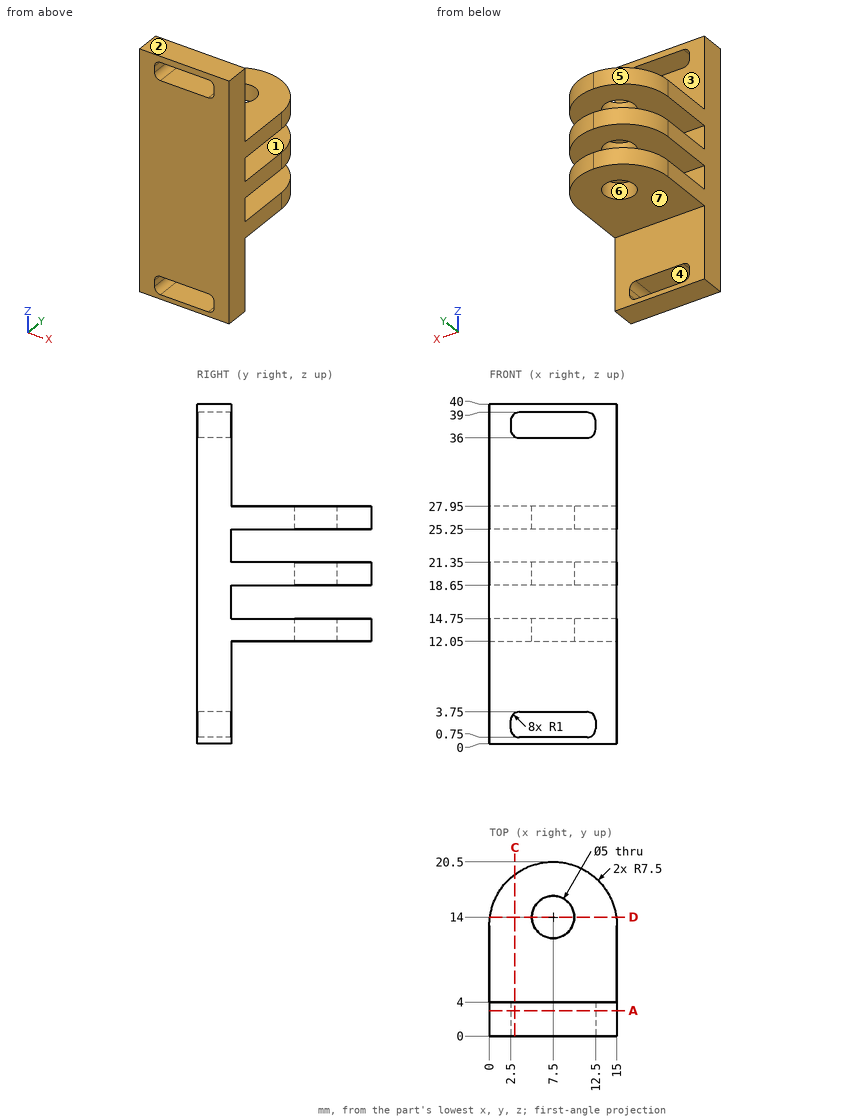
Here's the drawing with two shaded views (mm, measured from the low corner). I have some questions. A direction names the side the tool comes from. Coordinates: 2 decimals unless noted, no trailing zeros. Write each loop counter-clockwise with the first axis right and the second up, starting at its lowest first coordinate (ties: lowest second). Pieces come first, ordered by that corner, then holes. Notation, with made-up numbers: M 36.5,39 L 90.5,39 A26 cw 90.5,78 Z; hole C 54,18 d5. An arc over 180 degrees is marked long. Answer as CSV lines item,"result". Start each with the question number.
1) I want a section at A-A, the plane y = 3. Please give me the cut outline in (x, z), and give its area (3 significant figures).
2) I want a section at D-D, the plane y = 14. Please give me the cut outline in (x, z).
3) Please list where these lines run through material, in increasing order: line 1 (Z direction, x = 10.75, y = 11.25); line 2 (Y direction, x = 7.5, z = 19.3); line 3 (Y direction, x = 6.75, z = 8.5). Write a range as from..to.
4) For P1, Ø1.2, axis at x = 6, z = 24, coming from the +Y side; P2, Ø4, axis at x = 9.5, y = 14.5, coming from the +Z side; P3, Ø5, axis at x = 3.5, y = 14, coming from the -Z side, each with a flat end and sliding along its axis, tell me the tip position at first contact or that it passes through.
5) For the marked faces 1, 2, 3 and 4, which set-ups out of +Z, -Z, +X, -X, +Y, -Y let a thin tool reach every point of the face, with its end or its side?
6) I want a section at C-C, the plane x = 3. Please give me the cut outline in (y, z).
7) We'd pull the mould along X, two halves only. Please class the marked faces 5, 6 and 7: +X half, -X half, draft (parallel to the pull), parting line (faces both ways), or undercut.
Data:
1,outline,"M 0,0 L 15,0 L 15,40 L 0,40 Z; hole M 2.5,1.75 A1 ccw 3.5,0.75 L 11.5,0.75 A1 ccw 12.5,1.75 L 12.5,2.75 A1 ccw 11.5,3.75 L 3.5,3.75 A1 ccw 2.5,2.75 Z; hole M 2.5,37 A1 ccw 3.5,36 L 11.5,36 A1 ccw 12.5,37 L 12.5,38 A1 ccw 11.5,39 L 3.5,39 A1 ccw 2.5,38 Z"
1,area,"542 mm^2"
2,outline,"M 0.07,12.05 L 5,12.05 L 5,14.75 L 0.07,14.75 Z; M 0.07,18.65 L 5,18.65 L 5,21.35 L 0.07,21.35 Z; M 0.07,25.25 L 5,25.25 L 5,27.95 L 0.07,27.95 Z; M 10,12.05 L 14.93,12.05 L 14.93,14.75 L 10,14.75 Z; M 10,18.65 L 14.93,18.65 L 14.93,21.35 L 10,21.35 Z; M 10,25.25 L 14.93,25.25 L 14.93,27.95 L 10,27.95 Z"
3,line 1,"z = 12.05..14.75, 18.65..21.35, 25.25..27.95"
3,line 2,"y = 0..11.5, 16.5..20.5"
3,line 3,"y = 0..4"
4,P1,"stops at y = 4"
4,P2,"stops at z = 27.95"
4,P3,"stops at z = 12.05"
5,face 1,"+X, -X, +Y"
5,face 2,"+Z, +X, -X, +Y, -Y"
5,face 3,"+Z, +X, -X, +Y"
5,face 4,"+Y, -Y"
6,outline,"M 0,0 L 4,0 L 4,0.88 L 0,0.88 Z; M 0,3.62 L 4,3.62 L 4,12.05 L 19,12.05 L 19,14.75 L 4,14.75 L 4,18.65 L 19,18.65 L 19,21.35 L 4,21.35 L 4,25.25 L 19,25.25 L 19,27.95 L 4,27.95 L 4,36.13 L 0,36.13 Z; M 0,38.87 L 4,38.87 L 4,40 L 0,40 Z"
7,face 5,"-X half"
7,face 6,"undercut"
7,face 7,"draft"
